from build123d import *

# Parameters (mm, degrees)
AUFSATZ_LINEAR_AUSTRAGEN1_DEPTH = 30
SKIZZE2_R                       = 112.75
SKIZZE2_R_2                     = 89.75
SCHNITT_LINEAR_AUSTRAGEN1_DEPTH = 12
AUFSATZ_LINEAR_START            = 30
SKIZZE3_R                       = 125
AUFSATZ_LINEAR_AUSTRAGEN2_DEPTH = 30
SKIZZE4_W                       = 125
SKIZZE4_H                       = 28
SCHNITT_LINEAR_AUSTRAGEN2_DEPTH = 37


with BuildPart() as part:
    # Skizze1 → Aufsatz-Linear austragen1 (new body)
    with BuildSketch(Plane(origin=(0, 0, 0), x_dir=(1, 0, 0), z_dir=(0, 1, 0))):
        with BuildLine():
            ThreePointArc((0, 125), (-125, 0), (0, -125))
            Line((0, -125), (0, -112.75))
            ThreePointArc((0, -112.75), (-112.75, 0), (0, 112.75))
            Line((0, 112.75), (0, 125))
        make_face()
        with BuildLine():
            Line((0, -112.75), (0, -125))
            ThreePointArc((0, -125), (88.388347648, -88.388347648), (125, 0))
            ThreePointArc((125, 0), (88.388347648, 88.388347648), (0, 125))
            Line((0, 125), (0, 112.75))
            ThreePointArc((0, 112.75), (79.726289579, 79.726289579), (112.75, 0))
            ThreePointArc((112.75, 0), (79.726289579, -79.726289579), (0, -112.75))
        make_face()
        with BuildLine():
            ThreePointArc((0, 112.75), (-112.75, 0), (0, -112.75))
            Line((0, -112.75), (0, -89.75))
            ThreePointArc((0, -89.75), (-89.75, 0), (0, 89.75))
            Line((0, 89.75), (0, 112.75))
        make_face()
        with BuildLine():
            Line((0, -89.75), (0, -112.75))
            ThreePointArc((0, -112.75), (79.726289579, -79.726289579), (112.75, 0))
            ThreePointArc((112.75, 0), (79.726289579, 79.726289579), (0, 112.75))
            Line((0, 112.75), (0, 89.75))
            ThreePointArc((0, 89.75), (63.462833611, 63.462833611), (89.75, 0))
            ThreePointArc((89.75, 0), (63.462833611, -63.462833611), (0, -89.75))
        make_face()
        with BuildLine():
            ThreePointArc((0, 89.75), (-89.75, 0), (0, -89.75))
            Line((0, -89.75), (0, -75))
            ThreePointArc((0, -75), (-75, 0), (0, 75))
            Line((0, 75), (0, 89.75))
        make_face()
        with BuildLine():
            Line((0, -75), (0, -89.75))
            ThreePointArc((0, -89.75), (63.462833611, -63.462833611), (89.75, 0))
            ThreePointArc((89.75, 0), (63.462833611, 63.462833611), (0, 89.75))
            Line((0, 89.75), (0, 75))
            ThreePointArc((0, 75), (53.033008589, 53.033008589), (75, 0))
            ThreePointArc((75, 0), (53.033008589, -53.033008589), (0, -75))
        make_face()
    extrude(amount=AUFSATZ_LINEAR_AUSTRAGEN1_DEPTH)

    # Skizze2 → Schnitt-Linear austragen1 (cut)
    with BuildSketch(Plane(origin=(0, 30, 0), x_dir=(1, 0, 0), z_dir=(0, 1, 0))):
        with Locations(Location((0, 0, 0), (0, 0, 270))):
            Circle(SKIZZE2_R)
        with Locations(Location((0, 0, 0), (0, 0, 270))):
            Circle(SKIZZE2_R_2, mode=Mode.SUBTRACT)
    extrude(amount=-SCHNITT_LINEAR_AUSTRAGEN1_DEPTH, mode=Mode.SUBTRACT)

    # Skizze3 → Aufsatz-Linear austragen2 (add)
    # profile 1 of 5: a face of its own
    with BuildSketch(Plane.XZ.offset(AUFSATZ_LINEAR_START)):
        with Locations(Location((0, 0, 0), (0, 0, 90))):
            Circle(SKIZZE3_R)
        with BuildLine():
            Line((-88.388347648, -68.388347648), (-88.388347648, 68.388347648))
            ThreePointArc((-88.388347648, 68.388347648), (-82.530483272, 82.530483272), (-68.388347648, 88.388347648))
            Line((-68.388347648, 88.388347648), (68.388347648, 88.388347648))
            ThreePointArc((68.388347648, 88.388347648), (82.530483272, 82.530483272), (88.388347648, 68.388347648))
            Line((88.388347648, 68.388347648), (88.388347648, -68.388347648))
            ThreePointArc((88.388347648, -68.388347648), (82.530483272, -82.530483272), (68.388347648, -88.388347648))
            Line((68.388347648, -88.388347648), (-68.388347648, -88.388347648))
            ThreePointArc((-68.388347648, -88.388347648), (-82.530483272, -82.530483272), (-88.388347648, -68.388347648))
        make_face(mode=Mode.SUBTRACT)
    # profile 2 of 5: a face of its own
    with BuildSketch(Plane.XZ.offset(AUFSATZ_LINEAR_START)):
        with BuildLine():
            Line((-125, 125), (-125, 1.53e-07))
            ThreePointArc((-125, 1.53e-07), (-88.388347573, 88.388347723), (5.9e-08, 125))
            Line((5.9e-08, 125), (-125, 125))
        make_face()
    # profile 3 of 5: a face of its own
    with BuildSketch(Plane.XZ.offset(AUFSATZ_LINEAR_START)):
        with BuildLine():
            ThreePointArc((5.9e-08, 125), (88.388347669, 88.388347627), (125, 0))
            Line((125, 0), (125, 125))
            Line((125, 125), (5.9e-08, 125))
        make_face()
    # profile 4 of 5: a face of its own
    with BuildSketch(Plane.XZ.offset(AUFSATZ_LINEAR_START)):
        with BuildLine():
            ThreePointArc((125, 0), (88.388347702, -88.388347594), (1.52e-07, -125))
            Line((1.52e-07, -125), (125, -125))
            Line((125, -125), (125, 0))
        make_face()
    # profile 5 of 5: a face of its own
    with BuildSketch(Plane.XZ.offset(AUFSATZ_LINEAR_START)):
        with BuildLine():
            Line((-125, 1.53e-07), (-125, -125))
            Line((-125, -125), (1.52e-07, -125))
            ThreePointArc((1.52e-07, -125), (-88.388347648, -88.388347648), (-125, 1.53e-07))
        make_face()
    extrude(amount=-AUFSATZ_LINEAR_AUSTRAGEN2_DEPTH)

    # Skizze4 → Schnitt-Linear austragen2 (cut)
    with BuildSketch(Plane.XY.offset(125)):
        with Locations((0, -16)):
            Rectangle(SKIZZE4_W, SKIZZE4_H)
    extrude(amount=-SCHNITT_LINEAR_AUSTRAGEN2_DEPTH, mode=Mode.SUBTRACT)


solid = part.part
Geometry: final body of the model. Coordinates: model frame, mm. A direction names the side the tool comes from. Give positions to 0.01 mm unless a question says otherwise; leave off trailing zeros. Order: outer loops, then holes, each group sorted by start corner. A loop starts at its lowest first (then second) coordinate and runs counter-clockwise, first axis right, second up. Notation, with made-up numbers: (13.5, 19) -> (50.5, 19) arc R22 ccw to (50.5, 50) -> close; hole circle Ø7 at (89.5, 27.25). An arc over 180 degrees is marked (long way). Put each result on its own line as item: value.
Q1. Section A-A, the plane y = 25.5. Return loops of the section in (x, z), then the cut area to 3 significant figures.
Here are the results:
outline: circle Ø250 at (0, 0); circle Ø179.5 at (0, 0); hole circle Ø225.5 at (0, 0); hole circle Ø150 at (0, 0)
area: 16,800 mm^2
Q2. Material intervals for L1, parallel to Z at x = -64.5, y = -24.5; L2, parallel to X at y = 24, z = 14; L3, parallel to X at y = 27, z = 12, sorted ascending.
Here are the results:
L1: z = -125 to -88.39, 88.39 to 125
L2: x = -124.21 to -111.88, -88.65 to -73.68, 73.68 to 88.65, 111.88 to 124.21
L3: x = -124.42 to -112.11, -88.94 to -74.03, 74.03 to 88.94, 112.11 to 124.42
Q3. Pin query (flat end, axial travel): pin 1 (1.5 mm diameter, centred on x = 97, z = 38, fed in from +Y); pin 2 (3 mm diameter, centred on x = 65, y = 11.5, fed in from -Z); pin 3 (2 mm diameter, centred on x = -43.5, y = 3, fed in from +Z). Return the tip coordinate at first contact, or that it passes through.
Here are the results:
pin 1: stops at y = 18
pin 2: stops at z = -107.67
pin 3: stops at z = 117.55
Q4. Section B-B, the plane z = -49. Return loops of the section in (x, y).
Here are the results:
outline: (-125, -30) -> (-88.39, -30) -> (-88.39, 0) -> (-56.78, 0) -> (-56.78, 30) -> (-75.19, 30) -> (-75.19, 18) -> (-101.55, 18) -> (-101.55, 30) -> (-115, 30) -> (-115, 0) -> (-125, 0) -> close; (56.78, 0) -> (88.39, 0) -> (88.39, -30) -> (125, -30) -> (125, 0) -> (115, 0) -> (115, 30) -> (101.55, 30) -> (101.55, 18) -> (75.19, 18) -> (75.19, 30) -> (56.78, 30) -> close
Q5. Reachability of faces 3 (the face through (-100, 0, 95)), 4 (the face through (-87.616, 24.084, -19.456)), 5 (the face through (-100, 0, -95)), 6 (the face through (99, 0, -99)), 7 (the face through (82.37, -15.21, 82.69)) from +Z, -Z, +X, -X, +Y, -Y: full face, straight path, thin tool, end or side. Return the list, or none.
Here are the results:
face 3: +Z, -X, +Y
face 4: +Y
face 5: -Z, -X, +Y
face 6: -Z, +X, +Y
face 7: -Y
Q6. Section D-D, the plane y = -5. Return loops of the section in (x, z).
Here are the results:
outline: (-125, -125) -> (125, -125) -> (125, 125) -> (62.5, 125) -> (62.5, 88.39) -> (68.39, 88.39) arc R20 cw to (88.39, 68.39) -> (88.39, -68.39) arc R20 cw to (68.39, -88.39) -> (-68.39, -88.39) arc R20 cw to (-88.39, -68.39) -> (-88.39, 68.39) arc R20 cw to (-68.39, 88.39) -> (-62.5, 88.39) -> (-62.5, 125) -> (-125, 125) -> close
Q7. Draft query along Z for faces 1 (the face through (95, 0, 100)), 2 (the face through (-82.37, -15.21, -82.69)). Return one class per face: released by +Z, released by -Z, zero draft, split by the parting line, or undercut.
Here are the results:
face 1: zero draft
face 2: undercut
